from build123d import *

# Parameters (mm, degrees)
SKETCH1_W                                      = 25.4
SKETCH1_H                                      = 6.35
BOSS_EXTRUDE1_DEPTH                            = 6.35
CBORE_FOR_4_SOCKET_HEAD_CAP_SCREW1_D           = 3.2639
CBORE_FOR_4_SOCKET_HEAD_CAP_SCREW1_DEPTH       = 7.5946
CBORE_FOR_4_SOCKET_HEAD_CAP_SCREW1_CBORE_D     = 5.55752
CBORE_FOR_4_SOCKET_HEAD_CAP_SCREW1_CBORE_DEPTH = 2.8448
CBORE_FOR_4_SOCKET_HEAD_CAP_SCREW1_TIP         = 0.980574487
SKETCH4_R                                      = 3.7465
BOSS_EXTRUDE2_DEPTH                            = 5.715


with BuildPart() as part:
    # Sketch1 → Boss-Extrude1 (new body)
    with BuildSketch(Plane.XY):
        Rectangle(SKETCH1_W, SKETCH1_H)
    extrude(amount=BOSS_EXTRUDE1_DEPTH)

    # CBORE for _4 Socket Head Cap Screw1
    with Locations(Plane.XY.offset(6.35)):
        with Locations((-9.525, 0), (0, 0)):
            CounterBoreHole(CBORE_FOR_4_SOCKET_HEAD_CAP_SCREW1_D / 2, CBORE_FOR_4_SOCKET_HEAD_CAP_SCREW1_CBORE_D / 2, CBORE_FOR_4_SOCKET_HEAD_CAP_SCREW1_CBORE_DEPTH, depth=CBORE_FOR_4_SOCKET_HEAD_CAP_SCREW1_DEPTH)
            with Locations((0, 0, -(CBORE_FOR_4_SOCKET_HEAD_CAP_SCREW1_DEPTH + CBORE_FOR_4_SOCKET_HEAD_CAP_SCREW1_TIP / 2))):  # 118° drill point
                Cone(0, CBORE_FOR_4_SOCKET_HEAD_CAP_SCREW1_D / 2, CBORE_FOR_4_SOCKET_HEAD_CAP_SCREW1_TIP, mode=Mode.SUBTRACT)

    # Sketch4 → Boss-Extrude2 (add)
    with BuildSketch(Plane(origin=(12.7, -3.175, 6.35), x_dir=(0.40824829, -0.40824829, -0.816496581), z_dir=(0.577350269, -0.577350269, 0.577350269))):
        Circle(SKETCH4_R)
    extrude(amount=-BOSS_EXTRUDE2_DEPTH)


solid = part.part
For this review, take the finished solid that the model builds, in its own axes (mm). A direction names the side the tool comes from. Round coordinates to 2 decimals unless told otherwise and drop trailing zeros. Write each loop counter-clockwise with the first axis right and the second up, starting at its lowest first coordinate (ties: lowest second). Pieces come first, ordered by that corner, then holes. Notation, with made-up numbers: (69, 9.25) - (122, 9.25) arc R22 cw to (122, 41.25) - close; hole circle Ø6 at (54.5, 62). An arc over 180 degrees is marked (long way). Write item = value, one per line. Start each with the question number.
1. Consider section D-D on x = -10.25. State the section outline as (y, z) points (3 decimals).
2. For pin 1 Ø3 at (x, y) = (5.5, 0.5) entering from +Z; pin 2 Ø4 at (x, y) = (0, 0) entering from -Z; pin 3 Ø1.5 at (y, z) = (-4, 6.5) entering from +X, all flat-tipped, find the tip position at first contact; note any pin that passes through.
3. Draft analysis for pull direction X (two halves, no side actions). For faces 3 (the face through (12.7, 1, 1)), 4 (the face through (0, -2, 3.505)), 5 (the face through (0, 2, 0)), state which applies: released by +X, released by -X, zero draft, split by the parting line, or undercut.
4. Consider section C-C on z = 2.25. Give the number of separate pieces and of enclosed holes in the cut face, plus the area to 3 significant figures.
5. For faces 1 (the face through (-11.03, -0.63, 1.73)), 2 (the face through (-12.3, 0.1, 4.9)), list the 3-axis set-ups (+Z, -Z, +X, -X, +Y, -Y) from which the entire face can be reached by the end or side of a thin tool; tool diameter is ignored.
6. Consider section A-A on x = 0. State the section outline as (y, z) points (3 decimals), plus the area to 3 significant figures.
7. Consider section B-B on x = 4. State the section outline as (y, z) points (3 decimals), plus the area to 3 significant figures.
8. Wall thickness on L1, parallel to X at y = -2.25, z = 5.75 (3 decimals); L2, parallel to X at y = -1.25, z = 3; L3, parallel to Y at x = -3.5, z = 2.75 (3 decimals): over which ranges is each line inside the solid? List them lowest first.
Evaluation:
q1.outline = (-3.175, 0) - (-1.462, 0) - (-1.462, 3.505) - (-2.683, 3.505) - (-2.683, 6.35) - (-3.175, 6.35) - close; (1.462, 0) - (3.175, 0) - (3.175, 6.35) - (2.683, 6.35) - (2.683, 3.505) - (1.462, 3.505) - close
q2.pin_1 = 6.35
q2.pin_2 = 0
q2.pin_3 = 12.79
q3.face_3 = released by +X
q3.face_4 = undercut
q3.face_5 = zero draft
q4.separate_pieces = 1
q4.enclosed_holes = 2
q4.area = 154 mm2
q5.face_1 = +Z, -Z
q5.face_2 = +Z
q6.outline = (-3.175, 0) - (-1.632, 0) - (-1.632, 3.505) - (-2.779, 3.505) - (-2.779, 6.35) - (-3.175, 6.35) - close; (1.632, 0) - (3.175, 0) - (3.175, 6.35) - (2.779, 6.35) - (2.779, 3.505) - (1.632, 3.505) - close
q6.area = 13.1 mm2
q7.outline = (-3.175, 0) - (3.175, 0) - (3.175, 6.35) - (-3.175, 6.35) - close
q7.area = 40.3 mm2
q8.L1 = -12.7 to -11.156, -7.894 to -1.631, 1.631 to 14.225
q8.L2 = -12.7 to -10.57, -8.48 to -1.05, 1.05 to 14.48
q8.L3 = -3.175 to 3.175
